Source: CAD feature listing. Evaluate the final solid. Frame: model axes, mm. A direction names the side the tool comes from. Coordinates: 2 decimals unless noted, no trailing zeros. Loops run counter-clockwise (first coordinate to the right, second up) from the corner with the lowest first, then second, coordinate; pieces in that order, holes last. Notation, with made-up numbers: (-34, 26.5) - (3, 26.5) arc R31 ccw to (3, 58.5) - close; hole circle Ø2 at (32, 56.25). An arc over 180 degrees is marked (long way). Use CSV: the item, a comma, the result in double quotes. Start each with the question number.
```python
from build123d import *

# Parameters (mm, degrees)
SKETCH2_R               = 28.575
SKETCH2_R_2             = 3.2639
SKETCH2_R_3             = 52.3875
BOSS_EXTRUDE1_DEPTH     = 7.62
CUT_EXTRUDE1_DEPTH      = 369.60849746
CUT_EXTRUDE1_DEPTH_BACK = 369.60849746
SKETCH3_R               = 4.15
SKETCH3_R_2             = 2.5
CUT_EXTRUDE2_DEPTH      = 369.60849746
CUT_EXTRUDE2_DEPTH_BACK = 369.60849746


with BuildPart() as part:
    # Sketch2 → Boss-Extrude1 (new body)
    with BuildSketch(Plane.XY):
        with BuildLine():
            Line((-308.875210247, 91.684111495), (-215.925303767, 14.10662012))
            ThreePointArc((-215.925303767, 14.10662012), (-212.572234871, 12.65763879), (-208.970475069, 13.265869211))
            Line((-208.970475069, 13.265869211), (-134.814952137, 49.535152614))
            ThreePointArc((-134.814952137, 49.535152614), (-114.3, 46.0375), (-93.785047863, 49.535152614))
            Line((-93.785047863, 49.535152614), (-21.949808906, 13.301039962))
            ThreePointArc((-21.949808906, 13.301039962), (-14.699565425, 14.303090245), (-13.070560605, 21.438668609))
            Line((-13.070560605, 21.438668609), (-56.805390428, 130.917967399))
            ThreePointArc((-56.805390428, 130.917967399), (-79.093597182, 158.878055695), (-113.124724735, 169.851343962))
            Line((-113.124724735, 169.851343962), (-278.526789224, 172.991711242))
            ThreePointArc((-278.526789224, 172.991711242), (-322.495823899, 143.085706774), (-308.875210247, 91.684111495))
        make_face()
        with Locations(Location((-279.4, 127, 0), (0, 0, 180))):
            Circle(SKETCH2_R, mode=Mode.SUBTRACT)
        with Locations(Location((-19.05, 19.05, 0), (0, 0, 180))):
            Circle(SKETCH2_R_2, mode=Mode.SUBTRACT)
        with Locations(Location((-211.799479175, 19.05, 0), (0, 0, 180))):
            Circle(SKETCH2_R_2, mode=Mode.SUBTRACT)
        with Locations(Location((-114.3, 107.95, 0), (0, 0, 180))):
            Circle(SKETCH2_R_3, mode=Mode.SUBTRACT)
    extrude(amount=BOSS_EXTRUDE1_DEPTH)

    # Sketch3 → Cut-Extrude1 (cut, two sides: drawn at the far end of the back side and taken through both)
    with BuildSketch(Plane.XY.offset(7.62).offset(-CUT_EXTRUDE1_DEPTH_BACK)):
        with Locations((-279.4, 166.00043)):
            Circle(SKETCH3_R)
        with Locations((-254.746524018, 156.380868571)):
            Circle(SKETCH3_R)
        with Locations((-242.044200635, 133.164908097)):
            Circle(SKETCH3_R)
        with Locations((-247.236588134, 107.215554499)):
            Circle(SKETCH3_R)
        with Locations((-267.894110695, 90.674798722)):
            Circle(SKETCH3_R)
        with Locations((-294.35088393, 91.282244222)):
            Circle(SKETCH3_R)
        with Locations((-314.227489609, 108.753660501)):
            Circle(SKETCH3_R)
        with Locations((-318.223443029, 134.913977707)):
            Circle(SKETCH3_R)
        with Locations((-304.468993176, 157.522492681)):
            Circle(SKETCH3_R)
        with Locations((-114.3, 165.1)):
            Circle(SKETCH3_R_2)
        with Locations((-93.819271683, 161.304121374)):
            Circle(SKETCH3_R_2)
        with Locations((-74.960535999, 149.405145303)):
            Circle(SKETCH3_R_2)
        with Locations((-61.79108234, 130.509611392)):
            Circle(SKETCH3_R_2)
        with Locations((-57.15, 107.95)):
            Circle(SKETCH3_R_2)
        with Locations((-60.945878626, 87.469271683)):
            Circle(SKETCH3_R_2)
        with Locations((-72.844854697, 68.610535999)):
            Circle(SKETCH3_R_2)
        with Locations((-91.740388608, 55.44108234)):
            Circle(SKETCH3_R_2)
        with Locations((-114.3, 50.8)):
            Circle(SKETCH3_R_2)
        with Locations((-134.780728317, 54.595878626)):
            Circle(SKETCH3_R_2)
        with Locations((-153.639464001, 66.494854697)):
            Circle(SKETCH3_R_2)
        with Locations((-166.80891766, 85.390388608)):
            Circle(SKETCH3_R_2)
        with Locations((-171.45, 107.95)):
            Circle(SKETCH3_R_2)
        with Locations((-167.654121374, 128.430728317)):
            Circle(SKETCH3_R_2)
        with Locations((-155.755145303, 147.289464001)):
            Circle(SKETCH3_R_2)
        with Locations((-136.859611392, 160.45891766)):
            Circle(SKETCH3_R_2)
    extrude(amount=CUT_EXTRUDE1_DEPTH + CUT_EXTRUDE1_DEPTH_BACK, mode=Mode.SUBTRACT)

    # Sketch4 → Cut-Extrude2 (cut, two sides: drawn at the far end of the back side and taken through both)
    with BuildSketch(Plane.XY.offset(7.62).offset(-CUT_EXTRUDE2_DEPTH_BACK)):
        with BuildLine():
            Line((-278.860225121, 74.904185455), (-219.01939843, 24.960066172))
            ThreePointArc((-219.01939843, 24.960066172), (-217.078020776, 24.161494872), (-215.029526872, 24.620118947))
            ThreePointArc((-215.029526872, 24.620118947), (-211.026723478, 25.44236121), (-207.335161059, 23.689967346))
            ThreePointArc((-207.335161059, 23.689967346), (-205.454963796, 22.756414152), (-203.379217054, 23.069365873))
            Line((-203.379217054, 23.069365873), (-148.393096208, 49.962941986))
            ThreePointArc((-148.393096208, 49.962941986), (-146.441473652, 52.888826728), (-148.025123052, 56.029158988))
            ThreePointArc((-148.025123052, 56.029158988), (-167.202514386, 75.786641533), (-175.91672865, 101.90546472))
            ThreePointArc((-175.91672865, 101.90546472), (-177.022168822, 104.129423143), (-179.326246533, 105.05636162))
            Line((-179.326246533, 105.05636162), (-236.248291515, 106.1370986))
            ThreePointArc((-236.248291515, 106.1370986), (-238.04588498, 105.678406249), (-239.35496486, 104.363852787))
            ThreePointArc((-239.35496486, 104.363852787), (-255.112552192, 87.934415671), (-276.81836003, 81.072501319))
            ThreePointArc((-276.81836003, 81.072501319), (-279.937917376, 78.683040095), (-278.860225121, 74.904185455))
        make_face()
        with BuildLine():
            Line((-48.019318761, 91.807143198), (-22.303873454, 27.434904147))
            ThreePointArc((-22.303873454, 27.434904147), (-23.187455951, 23.564521405), (-27.120033775, 23.021003007))
            Line((-27.120033775, 23.021003007), (-80.387932313, 49.889641079))
            ThreePointArc((-80.387932313, 49.889641079), (-82.302626367, 52.822384958), (-80.709884678, 55.941714036))
            ThreePointArc((-80.709884678, 55.941714036), (-64.405072396, 71.294115674), (-54.62867895, 91.442695545))
            ThreePointArc((-54.62867895, 91.442695545), (-51.454892751, 93.998716793), (-48.019318761, 91.807143198))
        make_face()
        with BuildLine():
            Line((-243.572637688, 164.706689191), (-154.458722757, 163.014748867))
            ThreePointArc((-154.458722757, 163.014748867), (-151.211699304, 160.627169805), (-152.377082357, 156.768986628))
            ThreePointArc((-152.377082357, 156.768986628), (-168.115145357, 138.561889625), (-175.721811685, 115.729376938))
            ThreePointArc((-175.721811685, 115.729376938), (-176.902393858, 113.526279988), (-179.252929411, 112.6763429))
            Line((-179.252929411, 112.6763429), (-230.963872105, 113.658140516))
            ThreePointArc((-230.963872105, 113.658140516), (-233.622605418, 114.965574686), (-234.320208682, 117.845087947))
            ThreePointArc((-234.320208682, 117.845087947), (-235.210231249, 139.777493405), (-246.162459408, 158.800407158))
            ThreePointArc((-246.162459408, 158.800407158), (-246.837455621, 162.61732476), (-243.572637688, 164.706689191))
        make_face()
    extrude(amount=CUT_EXTRUDE2_DEPTH + CUT_EXTRUDE2_DEPTH_BACK, mode=Mode.SUBTRACT)


solid = part.part
```
(1) Reachability of faces 5 (the cylindrical face through (-82.3, 52.8, 3.8)), 6 (the flat face through (-58.37, 31.67, 3.76)), 7 (the cylindrical face through (-78.68, 158.59, 3.76)) from +Z, -Z, +X, -X, +Y, -Y: full face, straight path, thin tool, end or side. Return the list, or none.
(2) Section A-A on x = -125. Output: boundary loops of the cut face in (y, z).
(3) Draft query along Y for faces 1 (the cylindrical face through (-167.947, 138.856, 3.757)), 2 (the flat face through (-263.05, 53.44, 3.76)), 3 (the flat face through (-204, 111, 0)), 4 (the cylindrical face through (-322.21, 143.83, 3.76)). Return one class per face: released by +Y, released by -Y, zero draft, split by the parting line, or undercut.
(4) Section D-D on z = 4.5. State how many separate pieces and enclosed holes the cut face has, plus the area to 3 significant figures.
(5) Ray query, line 1 (X direction, y = 19.05, z = 4.5); line 2 (X direction, y = 41.5, z = 6.75); line 3 (Y direction, x = -161.5, z = 6.5). Return the intervals inside material, ascending. Write a range as [from, to].
(6) Section B-B on x = -305. Output: boundary loops of the cut face in (y, z), plus the area to 3 significant figures.
(7) Pin query (flat end, axial travel): pin 1 Ø5 at (x, y) = (-304.47, 157.52) entering from +Z; pin 2 Ø2 at (y, z) = (129, 2.5) entering from +X; pin 3 Ø3 at (x, z) = (-65.5, 2.5) entering from -Y; pin 4 Ø2 at (x, z) = (-269.5, 1) entering from +Y. Return the tip coordinate at first contact, or that it passes through.
(8) Section C-C on x = -19.05. Output: boundary loops of the cut face in (y, z).
Solution:
1,face 5,"+Z, -Z"
1,face 6,"+Z, -Z, -Y"
1,face 7,"+Z, -Z, +X, +Y"
2,outline,"(46.97, 0) - (56.67, 0) - (56.67, 7.62) - (46.97, 7.62) - close; (159.23, 0) - (170.08, 0) - (170.08, 7.62) - (159.23, 7.62) - close"
3,face 1,"undercut"
3,face 2,"released by -Y"
3,face 3,"zero draft"
3,face 4,"split by the parting line"
4,separate pieces,"1"
4,enclosed holes,"32"
4,area,"10,600 mm²"
5,line 1,"x = [-221.85, -215.06], [-208.54, -197.14], [-33.35, -22.31], [-15.79, -12.61]"
5,line 2,"x = [-248.75, -238.84], [-165.7, -151.24], [-77.86, -63.76], [-27.92, -21.08]"
5,line 3,"y = [36.48, 43.55], [67.88, 85.22], [130.68, 148.02], [163.15, 170.77]"
6,outline,"(88.45, 0) - (114.3, 0) - (114.3, 7.62) - (88.45, 7.62) - close; (139.7, 0) - (153.41, 0) - (153.41, 7.62) - (139.7, 7.62) - close; (161.64, 0) - (165.22, 0) - (165.22, 7.62) - (161.64, 7.62) - close"
6,area,"329 mm²"
7,pin 1,"passes through"
7,pin 2,"stops at x = -55.64"
7,pin 3,"stops at y = 34.51"
7,pin 4,"stops at y = 172.84"
8,outline,"(12.61, 0) - (15.79, 0) - (15.79, 7.62) - (12.61, 7.62) - close; (22.31, 0) - (36.41, 0) - (36.41, 7.62) - (22.31, 7.62) - close"
